from build123d import *

# Parameters (mm, degrees)
F0_W     = 76.2
F0_H     = 76.2
F1_DEPTH = 76.2
F2_R     = 5.08
F3_R     = 9.525
F4_DEPTH = 19.05
F5_SIZE  = 2.54
F6_R     = 9.525
F7_DEPTH = 19.05
F8_SIZE  = 2.54


with BuildPart() as f1:
    # F0 (on Top) → F1 (new body)
    with BuildSketch(Plane.XY):
        with Locations((0.757823, -1.647639)):
            Rectangle(F0_W, F0_H)
    extrude(amount=F1_DEPTH)

    # F2
    f2_edges = [f1.edges().sort_by_distance(p)[0] for p in [
        (-37.342177, -39.747639, 38.1),
        (38.857823, -39.747639, 38.1),
        (0.757823, -39.747639, 0),
        (0.757823, -39.747639, 76.2),
        (0.757823, 36.452361, 76.2),
        (-37.342177, -1.647639, 76.2),
        (38.857823, -1.647639, 76.2),
        (38.857823, 36.452361, 38.1),
        (38.857823, -1.647639, 0),
        (-37.342177, 36.452361, 38.1),
        (0.757823, 36.452361, 0),
        (-37.342177, -1.647639, 0),
    ]]
    fillet(f2_edges, radius=F2_R)

    # F3 (on face) → F4 (join)
    with BuildSketch(Plane(origin=(0, 36.452361, 0), x_dir=(-1, 0, 0), z_dir=(0, 1, 0))):
        with Locations((0, 38.857823)):
            Circle(F3_R)
    extrude(amount=F4_DEPTH)

    # F5
    f5_edges = [f1.edges().sort_by_distance(p)[0] for p in [
        (9.525, 55.502361, 38.857823),
    ]]
    chamfer(f5_edges, length=F5_SIZE)

    # F6 (on face) → F7 (join)
    with BuildSketch(Plane(origin=(-37.342177, 0, 0), x_dir=(0, -1, 0), z_dir=(-1, 0, 0))):
        with Locations((2.405462, 38.857823)):
            Circle(F6_R)
    extrude(amount=F7_DEPTH)

    # F8
    f8_edges = [f1.edges().sort_by_distance(p)[0] for p in [
        (-56.392177, 7.119538, 38.857823),
    ]]
    chamfer(f8_edges, length=F8_SIZE)


solid = f1.part
CAD build for the part. Positions are in the model's coordinates, mm. A direction names the side the tool comes from. Coordinates: 2 decimals unless noted, no trailing zeros. Write each loop counter-clockwise with the first axis right and the second up, starting at its lowest first coordinate (ties: lowest second). Pieces come first, ordered by that corner, then holes. Notation, with made-up numbers: M -30.5,7 L 22.5,7 A23 cw 22.5,29 Z; hole C 57.5,73.5 d6. An arc over 180 degrees is marked long. Answer as a JSON object with one key per item and string values. Group by question number.
1) Saw through at A-A (x = 0). Write the cut outline in (y, z).
2) Saw through at C-C (z = 63). Write the cut outline in (x, y).
3) Tool access for faces 1 (the face through (-35.894, -1.185, 74.672)), 2 (the face through (-37.342, 5, 30)), 3 (the face through (1.24, 44.59, 48.3)): list every direction of +Z, -Z, +X, -X, +Y, -Y with a clear straight run to the whole face (end or side of a thin tool).
4) Wall check: line 1 (Y direction, x = 24.5, z = 18); line 2 (X direction, y = -11, z = 15); line 3 (Z direction, x = -35, y = 19). Give the ranges that are in metal, low to high. Write a range as from..to.
5) Saw through at B-B (y = 19). Write the cut outline in (x, z).
6) Pin check, flat tips, straight feed: pin 1 Ø2 at (x, y) = (-14, 35) entering from -Z; pin 2 Ø8 at (y, z) = (-19, 50) entering from -X; pin 3 Ø3 at (x, y) = (-46, -10.5) entering from +Z. Stop position of each tip, or through.
Values follow:
{
 "1": {"outline": "M -39.75,5.08 A5.08 ccw -34.67,0 L 31.37,0 A5.08 ccw 36.45,5.08 L 36.45,29.33 L 52.96,29.33 L 55.5,31.87 L 55.5,45.84 L 52.96,48.38 L 36.45,48.38 L 36.45,71.12 A5.08 ccw 31.37,76.2 L -34.67,76.2 A5.08 ccw -39.75,71.12 Z"},
 "2": {"outline": "M -37.34,-34.67 A5.08 ccw -32.26,-39.75 L 33.78,-39.75 A5.08 ccw 38.86,-34.67 L 38.86,31.37 A5.08 ccw 33.78,36.45 L -32.26,36.45 A5.08 ccw -37.34,31.37 Z"},
 "3": {"face 1": "+Z, -X, +Y, -Y", "face 2": "-X", "face 3": "+Y"},
 "4": {"line 1": "y = -39.75..36.45", "line 2": "x = -37.34..38.86", "line 3": "z = 0.8..75.4"},
 "5": {"outline": "M -37.34,5.08 A5.08 ccw -32.26,0 L 33.78,0 A5.08 ccw 38.86,5.08 L 38.86,71.12 A5.08 ccw 33.78,76.2 L -32.26,76.2 A5.08 ccw -37.34,71.12 Z"},
 "6": {"pin 1": "stops at z = 0.73", "pin 2": "stops at x = -37.34", "pin 3": "stops at z = 45.73"}
}
